```python
from build123d import *

# Parameters (mm, degrees)
SKETCH_1_W      = 60
SKETCH_1_H      = 10
EXTRUDE_1_DEPTH = 1


with BuildPart() as part:
    # 草图1 → 凸台-拉伸1 (new body)
    with BuildSketch(Plane(origin=(0, 0, 0), x_dir=(0, 0, -1), z_dir=(1, 0, 0))):
        with Locations((28.433962264, 4.621952123)):
            Rectangle(SKETCH_1_W, SKETCH_1_H)
        with BuildLine():
            Line((3.433962264, 6.121952123), (53.433962264, 6.121952123))
            ThreePointArc((53.433962264, 6.121952123), (54.933962264, 4.621952123), (53.433962264, 3.121952123))
            Line((53.433962264, 3.121952123), (3.433962264, 3.121952123))
            ThreePointArc((3.433962264, 3.121952123), (1.933962264, 4.621952123), (3.433962264, 6.121952123))
        make_face(mode=Mode.SUBTRACT)
    extrude(amount=EXTRUDE_1_DEPTH)


solid = part.part
```
Could you check a few things on this model? Use its own coordinates, in mm. A direction names the side the tool comes from. Round coordinates to 2 decimals unless told otherwise and drop trailing zeros. Loops run counter-clockwise (first coordinate to the right, second up) from the corner with the lowest first, then second, coordinate; pieces in that order, holes last. Notation, with made-up numbers: (-27.5, -17.75) -> (-18.5, -17.75) arc R20 cw to (-18.5, -0.75) -> close; hole circle Ø9 at (23, 8.5). An arc over 180 degrees is marked (long way). One line per question, with ' | ' between items.
(1) For faces 4 (the face through (0.5, 4.6, 1.566)), 5 (the face through (0.5, 3.122, -28.8)), which set-ups out of +Z, -Z, +X, -X, +Y, -Y let a thin tool reach every point of the face, with its end or its side?
Model answer:
face 4: +Z, +X, -X, +Y, -Y | face 5: +X, -X
(2) If we section it at C-C on y = 4.25: List the corners of the cut face in (x, z) for me.
Model answer:
outline: (0, -58.43) -> (1, -58.43) -> (1, -54.89) -> (0, -54.89) -> close; (0, -1.98) -> (1, -1.98) -> (1, 1.57) -> (0, 1.57) -> close
(3) If we section it at A-A on z = -30.5: List the corners of the cut face in (x, y) for me.
Model answer:
outline: (0, -0.38) -> (1, -0.38) -> (1, 3.12) -> (0, 3.12) -> close; (0, 6.12) -> (1, 6.12) -> (1, 9.62) -> (0, 9.62) -> close
(4) If we section it at B-B on x = 0.6: List the corners of the cut face in (y, z) for me, and give its area (3 significant figures).
Model answer:
outline: (-0.38, -58.43) -> (9.62, -58.43) -> (9.62, 1.57) -> (-0.38, 1.57) -> close; hole (3.12, -53.43) arc R1.5 ccw to (6.12, -53.43) -> (6.12, -3.43) arc R1.5 ccw to (3.12, -3.43) -> close | area: 443 mm^2
(5) If I drill on probe 1 along Y at (x, z) = (0.9, -47.5); probe 2 along Z at (x, y) = (0.4, 4.75); probe 3 along Z at (x, y) = (0.3, 5.5), over which ranges is the centre line in solid material (lowest first)?
Model answer:
probe 1: y = -0.38 to 3.12, 6.12 to 9.62 | probe 2: z = -58.43 to -54.93, -1.94 to 1.57 | probe 3: z = -58.43 to -54.65, -2.22 to 1.57
(6) Thinking about a two-plate mould opening in Y: for faces 1 (the face through (0.5, -0.378, -28)), 2 (the face through (0, 7, -28)), 3 (the face through (0.493, 4.589, -1.934)), which applies, released by +Y, released by -Y, zero draft, split by the parting line, or undercut?
Model answer:
face 1: released by -Y | face 2: zero draft | face 3: undercut
